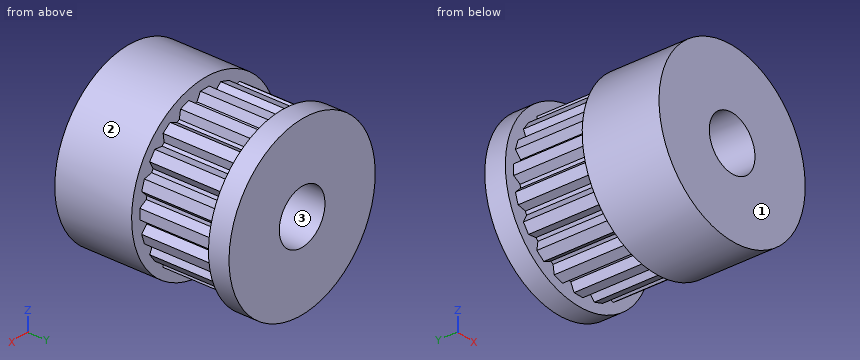
from build123d import *

# Parameters (mm, degrees)
SKETCH1_R               = 8
BOSS_EXTRUDE1_DEPTH     = 7.1
BOSS_EXTRUDE2_DEPTH     = 7.1
SKETCH3_R               = 8
BOSS_EXTRUDE3_DEPTH     = 1.9
CUT_EXTRUDE1_DEPTH      = 20.677652299
CUT_EXTRUDE1_DEPTH_BACK = 20.677652299
SKETCH4_R               = 2.5


with BuildPart() as part:
    # Sketch1 → Boss-Extrude1 (new body)
    with BuildSketch(Plane(origin=(0, 0, 0), x_dir=(1, 0, 0), z_dir=(0, 1, 0))):
        with Locations(Location((0, 0, 0), (0, 0, 270))):
            Circle(SKETCH1_R)
    extrude(amount=BOSS_EXTRUDE1_DEPTH)

    # Sketch2 → Boss-Extrude2 (add)
    with BuildSketch(Plane(origin=(0, 7.1, 0), x_dir=(1, 0, 0), z_dir=(0, 1, 0))):
        with BuildLine():
            Line((-0.475669396, 7.098967945), (-0.844267822, 6.384436135))
            ThreePointArc((-0.844267822, 6.384436135), (-0.992920102, 6.363012069), (-1.14103236, 6.338127332))
            Line((-1.14103236, 6.338127332), (-1.741313259, 6.89850965))
            Line((-1.741313259, 6.89850965), (-2.646090217, 6.604529796))
            Line((-2.646090217, 6.604529796), (-2.775845679, 5.811066484))
            ThreePointArc((-2.775845679, 5.811066484), (-2.90801175, 5.739642443), (-3.043775319, 5.675318909))
            Line((-3.043775319, 5.675318909), (-3.78784404, 6.022777166))
            Line((-3.78784404, 6.022777166), (-4.55749329, 5.463594254))
            Line((-4.55749329, 5.463594254), (-4.43570442, 4.668869158))
            ThreePointArc((-4.43570442, 4.668869158), (-4.545755036, 4.566553145), (-4.648572343, 4.45697073))
            Line((-4.648572343, 4.45697073), (-5.463594254, 4.557493289))
            Line((-5.463594254, 4.557493289), (-6.022777166, 3.787844039))
            Line((-6.022777166, 3.787844039), (-5.661365507, 3.069650389))
            ThreePointArc((-5.661365507, 3.069650389), (-5.74260171, 2.942530762), (-5.798334717, 2.802343202))
            Line((-5.798334717, 2.802343202), (-6.604529796, 2.646090216))
            Line((-6.604529796, 2.646090216), (-6.89850965, 1.741313258))
            Line((-6.89850965, 1.741313258), (-6.332852694, 1.169952852))
            ThreePointArc((-6.332852694, 1.169952852), (-6.358413277, 1.021955731), (-6.38051569, 0.873402797))
            Line((-6.38051569, 0.873402797), (-7.098967945, 0.475669396))
            Line((-7.098967945, 0.475669396), (-7.098967945, -0.475669396))
            Line((-7.098967945, -0.475669396), (-6.384436135, -0.844267822))
            ThreePointArc((-6.384436135, -0.844267822), (-6.363012069, -0.992920102), (-6.338127332, -1.14103236))
            Line((-6.338127332, -1.14103236), (-6.89850965, -1.741313259))
            Line((-6.89850965, -1.741313259), (-6.604529796, -2.646090217))
            Line((-6.604529796, -2.646090217), (-5.811066484, -2.775845679))
            ThreePointArc((-5.811066484, -2.775845679), (-5.744754906, -2.910601998), (-5.675318909, -3.043775319))
            Line((-5.675318909, -3.043775319), (-6.022777166, -3.78784404))
            Line((-6.022777166, -3.78784404), (-5.463594254, -4.55749329))
            Line((-5.463594254, -4.55749329), (-4.668869158, -4.43570442))
            ThreePointArc((-4.668869158, -4.43570442), (-4.564161106, -4.543373891), (-4.45697073, -4.648572343))
            Line((-4.45697073, -4.648572343), (-4.557493289, -5.463594254))
            Line((-4.557493289, -5.463594254), (-3.787844039, -6.022777166))
            Line((-3.787844039, -6.022777166), (-3.069650389, -5.661365507))
            ThreePointArc((-3.069650389, -5.661365507), (-2.936795417, -5.731408691), (-2.802343202, -5.798334717))
            Line((-2.802343202, -5.798334717), (-2.646090216, -6.604529796))
            Line((-2.646090216, -6.604529796), (-1.741313258, -6.89850965))
            Line((-1.741313258, -6.89850965), (-1.169952852, -6.332852694))
            ThreePointArc((-1.169952852, -6.332852694), (-1.021955731, -6.358413277), (-0.873402797, -6.38051569))
            Line((-0.873402797, -6.38051569), (-0.475669396, -7.098967945))
            Line((-0.475669396, -7.098967945), (0.475669396, -7.098967945))
            Line((0.475669396, -7.098967945), (0.844267822, -6.384436135))
            ThreePointArc((0.844267822, -6.384436135), (0.992920102, -6.363012069), (1.14103236, -6.338127332))
            Line((1.14103236, -6.338127332), (1.741313259, -6.89850965))
            Line((1.741313259, -6.89850965), (2.646090217, -6.604529796))
            Line((2.646090217, -6.604529796), (2.775845679, -5.811066484))
            ThreePointArc((2.775845679, -5.811066484), (2.910601998, -5.744754906), (3.043775319, -5.675318909))
            Line((3.043775319, -5.675318909), (3.78784404, -6.022777166))
            Line((3.78784404, -6.022777166), (4.55749329, -5.463594254))
            Line((4.55749329, -5.463594254), (4.43570442, -4.668869158))
            ThreePointArc((4.43570442, -4.668869158), (4.543373891, -4.564161106), (4.648572343, -4.45697073))
            Line((4.648572343, -4.45697073), (5.463594254, -4.557493289))
            Line((5.463594254, -4.557493289), (6.022777166, -3.787844039))
            Line((6.022777166, -3.787844039), (5.661365507, -3.069650389))
            ThreePointArc((5.661365507, -3.069650389), (5.73140869, -2.936795416), (5.798334717, -2.802343202))
            Line((5.798334717, -2.802343202), (6.604529796, -2.646090216))
            Line((6.604529796, -2.646090216), (6.89850965, -1.741313258))
            Line((6.89850965, -1.741313258), (6.332852694, -1.169952852))
            ThreePointArc((6.332852694, -1.169952852), (6.358413277, -1.021955731), (6.38051569, -0.873402797))
            Line((6.38051569, -0.873402797), (7.098967945, -0.475669396))
            Line((7.098967945, -0.475669396), (7.098967945, 0.475669396))
            Line((7.098967945, 0.475669396), (6.384436135, 0.844267822))
            ThreePointArc((6.384436135, 0.844267822), (6.363012069, 0.992920102), (6.338127332, 1.14103236))
            Line((6.338127332, 1.14103236), (6.89850965, 1.741313259))
            Line((6.89850965, 1.741313259), (6.604529796, 2.646090217))
            Line((6.604529796, 2.646090217), (5.819778459, 2.774421005))
            ThreePointArc((5.819778459, 2.774421005), (5.755101615, 2.913148935), (5.675318909, 3.043775319))
            Line((5.675318909, 3.043775319), (6.022777166, 3.78784404))
            Line((6.022777166, 3.78784404), (5.463594254, 4.55749329))
            Line((5.463594254, 4.55749329), (4.668869158, 4.43570442))
            ThreePointArc((4.668869158, 4.43570442), (4.564161105, 4.54337389), (4.45697073, 4.648572343))
            Line((4.45697073, 4.648572343), (4.557493289, 5.463594254))
            Line((4.557493289, 5.463594254), (3.787844039, 6.022777166))
            Line((3.787844039, 6.022777166), (3.069650389, 5.661365507))
            ThreePointArc((3.069650389, 5.661365507), (2.936795417, 5.731408691), (2.802343202, 5.798334717))
            Line((2.802343202, 5.798334717), (2.646090216, 6.604529796))
            Line((2.646090216, 6.604529796), (1.741313258, 6.89850965))
            Line((1.741313258, 6.89850965), (1.169952852, 6.332852694))
            Line((1.169952852, 6.332852694), (0.873402797, 6.38051569))
            Line((0.873402797, 6.38051569), (0.475669396, 7.098967945))
            Line((0.475669396, 7.098967945), (-0.475669396, 7.098967945))
        make_face()
    extrude(amount=BOSS_EXTRUDE2_DEPTH)

    # Sketch3 → Boss-Extrude3 (add)
    with BuildSketch(Plane(origin=(0, 14.2, 0), x_dir=(1, 0, 0), z_dir=(0, 1, 0))):
        with Locations(Location((0, 0, 0), (0, 0, 270))):
            Circle(SKETCH3_R)
    extrude(amount=BOSS_EXTRUDE3_DEPTH)

    # Sketch4 → Cut-Extrude1 (cut, two sides: drawn at the far end of the back side and taken through both)
    with BuildSketch(Plane(origin=(0, 16.1, 0), x_dir=(1, 0, 0), z_dir=(0, 1, 0)).offset(-CUT_EXTRUDE1_DEPTH_BACK)):
        with Locations(Location((0, 0, 0), (0, 0, 270))):
            Circle(SKETCH4_R)
    extrude(amount=CUT_EXTRUDE1_DEPTH + CUT_EXTRUDE1_DEPTH_BACK, mode=Mode.SUBTRACT)


solid = part.part
Can you work these out from the model? Positions are in its coordinate system, mm. Face numbers are marked on the shaded views. Give positions to 0.01 mm unless a question says otherwise; leave off trailing zeros. Write each loop counter-clockwise with the first axis right and the second up, starting at its lowest first coordinate (ties: lowest second). Pieces come first, ordered by that corner, then holes. Notation, with made-up numbers: M -39.75,-16.5 L 15.25,-16.5 A18 ccw 15.25,9.5 Z; hole C -37.5,24 d8. An arc over 180 degrees is marked long. Answer in a Markdown table with one row per item. Add a question column.
Item 1: Imagine slicing it at C-C, the plane y = 15. Write out the boundary of the cut face in (x, z).
Item 2: Please list where these lines run through material, in increasing order: L1, parallel to Y at x = -6.25, z = -4.75; L2, parallel to X at y = 11.5, z = 0; L3, parallel to X at y = 5.5, z = 0.
Item 3: Imagine slicing it at B-B, the plane x = 0. Write out the boundary of the cut face in (y, z), plus the area to 3 significant figures.
Item 4: We'd pull the mould along X, two halves only. Please class the marked faces 1, 2 and 3: released by +X, released by -X, zero draft, split by the parting line, or undercut.
Item 5: For pin 1 Ø1 at (y, z) = (9.5, 0) entering from -X; pin 2 Ø1 at (y, z) = (9, 0) entering from +X; pin 3 Ø5 at (y, z) = (5, 6) entering from +X, each with a flat end and sliding along its axis, tell me the tip position at first contact or that it passes through.
Item 6: Imagine slicing it at A-A, the plane z = 0. Write out the boundary of the cut face in (x, y), plus the area to 3 significant figures.
Evaluation:
| question | item | result |
|---|---|---|
| 1 | outline | C 0,0 d16; hole C 0,0 d5 |
| 2 | L1 | y = 0 to 7.1, 14.2 to 16.1 |
| 2 | L2 | x = -7.1 to -2.5, 2.5 to 7.1 |
| 2 | L3 | x = -8 to -2.5, 2.5 to 8 |
| 3 | outline | M 0,-8 L 7.1,-8 L 7.1,-7.1 L 14.2,-7.1 L 14.2,-8 L 16.1,-8 L 16.1,-2.5 L 0,-2.5 Z; M 0,2.5 L 16.1,2.5 L 16.1,8 L 14.2,8 L 14.2,7.1 L 7.1,7.1 L 7.1,8 L 0,8 Z |
| 3 | area | 164 mm² |
| 4 | face 1 | zero draft |
| 4 | face 2 | split by the parting line |
| 4 | face 3 | undercut |
| 5 | pin 1 | stops at x = -7.1 |
| 5 | pin 2 | stops at x = 7.1 |
| 5 | pin 3 | stops at x = 7.19 |
| 6 | outline | M -8,0 L -2.5,0 L -2.5,16.1 L -8,16.1 L -8,14.2 L -7.1,14.2 L -7.1,7.1 L -8,7.1 Z; M 2.5,0 L 8,0 L 8,7.1 L 7.1,7.1 L 7.1,14.2 L 8,14.2 L 8,16.1 L 2.5,16.1 Z |
| 6 | area | 164 mm² |
